The figure shows three views and two pictorial views of one solid part (mm, origin at its lowest corner). Answer the questions. Round coordinates to 2 decimals unless told otherwise and drop trailing zeros. Order: outer loops, then holes, each group sorted by start corner. A loop starts at its lowest first (then second) coordinate and runs counter-clockwise, first axis right, second up. Notation, with made-up numbers: (-22.75, -4) -> (22.25, -4) arc R22 ccw to (22.25, 27) -> close; hole circle Ø2 at (27.25, 80.5). An arc over 180 degrees is marked (long way). One line per item, written item: value. Start each with the question number.
1. Section C-C (y = 1.75) is taken. Give the vertices of the cut face in (x, z), then the cut area to 3 significant figures.
2. Section B-B (z = 89) is taken. Give the vertices of the cut face in (x, y), then the cut area to 3 significant figures.
3. Consider line 1 (Z direction, x = 35, y = 2.35); line 2 (Z direction, x = 61.5, y = 0.5); line 3 (Z direction, x = 63, y = 2.5). Determine where each line is inside the solid, lowest interval first.
4. Section A-A (x = 35) is taken. Give the vertices of the cut face in (y, z), then the cut area to 3 significant figures.
5. Section D-D (x = 6) is taken. Give the vertices of the cut face in (y, z), then the cut area to 3 significant figures.
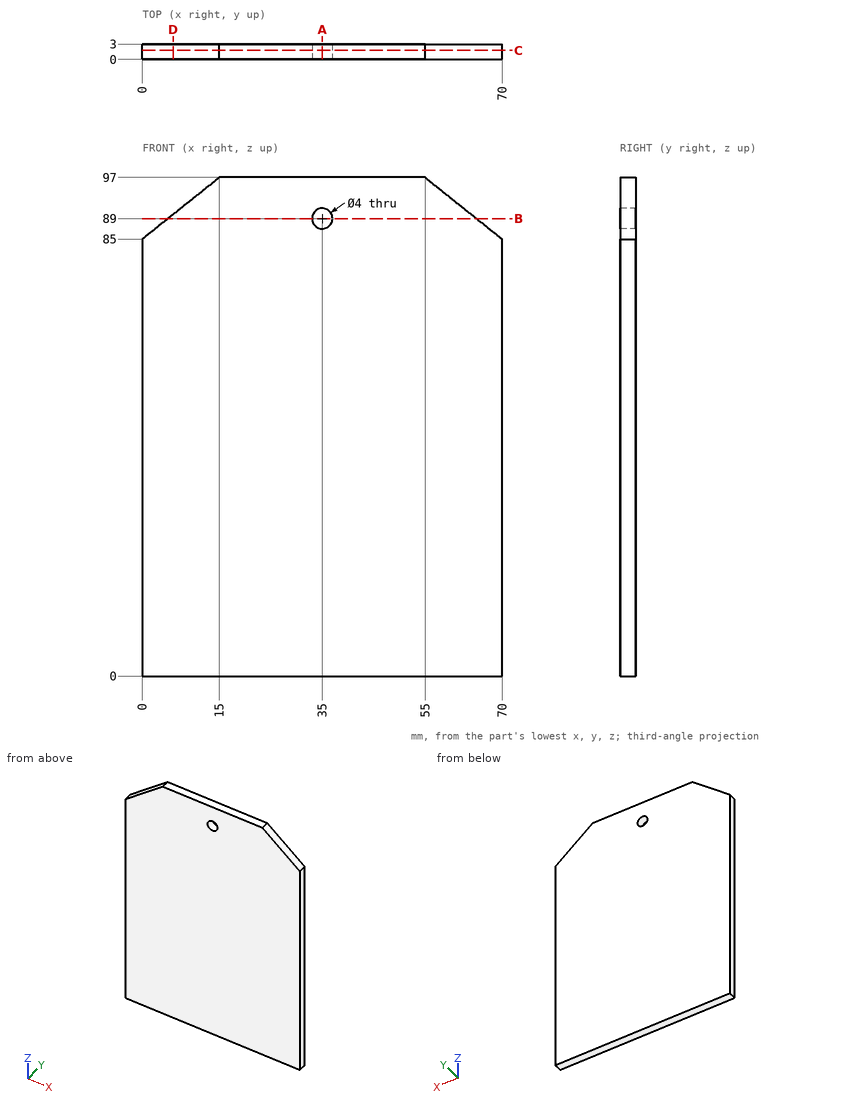
Answer:
1. outline: (0, 0) -> (70, 0) -> (70, 85) -> (55, 97) -> (15, 97) -> (0, 85) -> close; hole circle Ø4 at (35, 89)
1. area: 6,600 mm^2
2. outline: (5, 0) -> (33, 0) -> (33, 3) -> (5, 3) -> close; (37, 0) -> (65, 0) -> (65, 3) -> (37, 3) -> close
2. area: 168 mm^2
3. line 1: 0 to 87, 91 to 97
3. line 2: 0 to 91.8
3. line 3: 0 to 90.6
4. outline: (0, 0) -> (3, 0) -> (3, 87) -> (0, 87) -> close; (0, 91) -> (3, 91) -> (3, 97) -> (0, 97) -> close
4. area: 279 mm^2
5. outline: (0, 0) -> (3, 0) -> (3, 89.8) -> (0, 89.8) -> close
5. area: 269 mm^2
